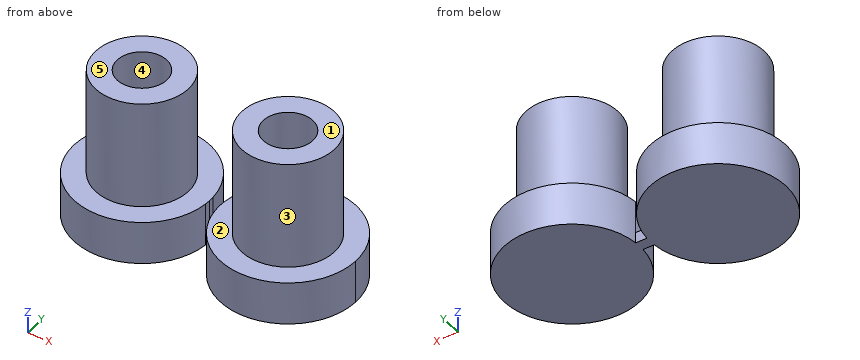
from build123d import *

# Parameters (mm, degrees)
F0_R     = 2.15
F0_R_2   = 1.15
F1_DEPTH = 7
F2_DEPTH = 2
F3_DEPTH = 0.5


with BuildPart() as f1:
    # F0 (on Top) → F1 (new body)
    with BuildSketch(Plane.XY):
        with Locations((-25.0254408006, 19.4505679031)):
            Circle(F0_R)
        with Locations((-25.0254408006, 19.4505679031)):
            Circle(F0_R_2, mode=Mode.SUBTRACT)
    extrude(amount=F1_DEPTH)

    # F0 (on Top) → F2 (join)
    with BuildSketch(Plane.XY):
        with BuildLine():
            ThreePointArc((-21.8856664985, 19.1969592827), (-21.8779982633, 19.3236605577), (-21.8754408006, 19.4505679031))
            ThreePointArc((-21.8754408006, 19.4505679031), (-21.8779982633, 19.5774752484), (-21.8856664985, 19.7041765234))
            ThreePointArc((-21.8856664985, 19.7041765234), (-28.1754408006, 19.4505679031), (-21.8856664985, 19.1969592827))
        make_face()
        with Locations((-25.0254408006, 19.4505679031)):
            Circle(F0_R, mode=Mode.SUBTRACT)
        with Locations((-25.0254408006, 19.4505679031)):
            Circle(F0_R_2)
    extrude(amount=F2_DEPTH)



with BuildPart() as f1b:
    # F0 (on Top) → F1, piece 2 (new body)
    with BuildSketch(Plane.XY):
        with Locations((-18.2254408006, 19.4505679031)):
            Circle(F0_R)
        with Locations((-18.2254408006, 19.4505679031)):
            Circle(F0_R_2, mode=Mode.SUBTRACT)
    extrude(amount=F1_DEPTH)

    # F0 (on Top) → F2, piece 2 (join)
    with BuildSketch(Plane.XY):
        with BuildLine():
            ThreePointArc((-15.0754408006, 19.4505679031), (-18.0985334552, 22.5980104404), (-21.3652151026, 19.7041765234))
            ThreePointArc((-21.3652151026, 19.7041765234), (-21.3754408006, 19.4505679031), (-21.3652151026, 19.1969592827))
            ThreePointArc((-21.3652151026, 19.1969592827), (-18.0985334552, 16.3031253657), (-15.0754408006, 19.4505679031))
        make_face()
        with Locations((-18.2254408006, 19.4505679031)):
            Circle(F0_R, mode=Mode.SUBTRACT)
        with Locations((-18.2254408006, 19.4505679031)):
            Circle(F0_R_2)
    extrude(amount=F2_DEPTH)


with BuildPart() as f1_1:
    add(f1.part)

    add(f1b.part)  # F3 merges F1b
    # F0 (on Top) → F3 (join)
    with BuildSketch(Plane.XY):
        with BuildLine():
            ThreePointArc((-21.8856664985, 19.7041765234), (-21.8779982633, 19.5774752484), (-21.8754408006, 19.4505679031))
            ThreePointArc((-21.8754408006, 19.4505679031), (-21.8779982633, 19.3236605577), (-21.8856664985, 19.1969592827))
            Line((-21.8856664985, 19.1969592827), (-21.3652151026, 19.1969592827))
            ThreePointArc((-21.3652151026, 19.1969592827), (-21.3754408006, 19.4505679031), (-21.3652151026, 19.7041765234))
            Line((-21.3652151026, 19.7041765234), (-21.8856664985, 19.7041765234))
        make_face()
    extrude(amount=F3_DEPTH)


solid = f1_1.part
Read the model definition and answer for the solid it produces. Units are mm, in the model's axes. Face numbers are marked on the shaded views. A direction names the side the tool comes from. Give positions to 0.01 mm unless a question says otherwise; leave off trailing zeros. Loops run counter-clockwise (first coordinate to the right, second up) from the corner with the lowest first, then second, coordinate; pieces in that order, holes last. Notation, with made-up numbers: (-9, 80) - (35, 80) arc R34 cw to (35, 113) - close; hole circle Ø2 at (-25, -6.75). An arc over 180 degrees is marked (long way). Answer as CSV lines item,"result". Start each with the question number.
1) Each of these flat-tipped pins is pushed along its axis until it touches: pin 1 Ø0.6 at (x, y) = (-22, 19.5) entering from +Z; pin 2 Ø1 at (y, z) = (18, 1) entering from +X; pin 3 Ø2 at (x, z) = (-21.5, 5.5) entering from +Y. Where does it stop, or does it pass through?
2) Determine the mould class of the marked faces 3, 4 and 5 for opening direction Y: released by +Y, released by -Y, zero draft, split by the parting line, or undercut.
3) Find section D-D (x = -26). Write down the section's boundary in (y, z).
4) Find section A-A (z = 1.5). Write down the section's boundary in (x, y), then the cut area to 3 significant figures.
5) Straight lines are drawn through the part: L1, parallel to X at y = 19.5, z = 2.25; L2, parallel to X at y = 18.75, z = 3.25; L3, parallel to Y at x = -25, z = 5.25. For each, find the intervals that lie inside material, in ascending order. Write a range as from..to.
6) Find section C-C (z = 6). Write down the section's boundary in (x, y), then the cut area to 3 significant figures.
7) Find section B-B (y = 18). Write down the section's boundary in (x, z).
8) Which of the six approach directions +Z, -Z, +X, -X, +Y, -Y give full straight-line access (tool end or side, diameter ignored) to the marked faces 1 and 2?
Findings below:
1,pin 1,"z = 2"
1,pin 2,"x = -15.22"
1,pin 3,"through"
2,face 3,"split by the parting line"
2,face 4,"undercut"
2,face 5,"zero draft"
3,outline,"(16.46, 0) - (22.45, 0) - (22.45, 2) - (21.37, 2) - (21.37, 7) - (20.06, 7) - (20.06, 2) - (18.84, 2) - (18.84, 7) - (17.53, 7) - (17.53, 2) - (16.46, 2) - close"
4,outline,"circle Ø6.3 at (-25.03, 19.45); circle Ø6.3 at (-18.23, 19.45)"
4,area,"62.3 mm^2"
5,L1,"-27.17..-26.17, -23.88..-22.88, -20.37..-19.37, -17.08..-16.08"
5,L2,"-27.06..-25.94, -24.11..-22.99, -20.26..-19.14, -17.31..-16.19"
5,L3,"17.3..18.3, 20.6..21.6"
6,outline,"circle Ø4.3 at (-25.03, 19.45); circle Ø4.3 at (-18.23, 19.45); hole circle Ø2.3 at (-25.03, 19.45); hole circle Ø2.3 at (-18.23, 19.45)"
6,area,"20.7 mm^2"
7,outline,"(-27.82, 0) - (-22.23, 0) - (-22.23, 2) - (-23.44, 2) - (-23.44, 7) - (-26.61, 7) - (-26.61, 2) - (-27.82, 2) - close; (-21.02, 0) - (-15.43, 0) - (-15.43, 2) - (-16.64, 2) - (-16.64, 7) - (-19.81, 7) - (-19.81, 2) - (-21.02, 2) - close"
8,face 1,"+Z, +X, -X, +Y, -Y"
8,face 2,"+Z"
